Here's how the part is built. I have some questions about the finished solid (model axes, mm). A direction names the side the tool comes from. Give positions to 0.01 mm unless a question says otherwise; leave off trailing zeros.
from build123d import *

# Parameters (mm, degrees)
SKETCH1_R           = 2.5
BOSS_EXTRUDE1_DEPTH = 13.97
CUT_EXTRUDE1_REACH  = 108.146
SKETCH2_R           = 2.5
FILLET1_R           = 5
FILLET2_R           = 1


with BuildPart() as part:
    # Sketch1 → Boss-Extrude1 (new body)
    with BuildSketch(Plane(origin=(0, 0, 0), x_dir=(1, 0, 0), z_dir=(0, 1, 0))):
        Polygon((0, 7.071067812), (-7.071067812, 0), (62.778932188, -69.85), (81.2, -69.85), (81.2, -59.85), (66.921067812, -59.85), align=None)
        with Locations(Location((0, 0, 0), (0, 0, 270))):
            Circle(SKETCH1_R, mode=Mode.SUBTRACT)
    extrude(amount=BOSS_EXTRUDE1_DEPTH)

    # Sketch2 → Cut-Extrude1 (cut, up to next)
    with BuildSketch(Plane(origin=(0, 0, 59.85), x_dir=(-1, 0, 0), z_dir=(0, 0, -1)), mode=Mode.PRIVATE) as cut_extrude1_sk1:
        with Locations((-76.2, 7.62)):
            Circle(SKETCH2_R)
    cut_extrude1_tool1 = extrude(cut_extrude1_sk1.sketch, amount=-CUT_EXTRUDE1_REACH, mode=Mode.PRIVATE) & part.part
    add(cut_extrude1_tool1.solids().sort_by_distance((76.2, 7.62, 59.85))[0], mode=Mode.SUBTRACT)

    # Fillet1
    fillet1_edges = [part.edges().sort_by_distance(p)[0] for p in [
        (0, 6.985, -7.071067812),
        (-7.071067812, 6.985, 0),
        (81.2, 0, 64.85),
        (81.2, 13.97, 64.85),
        (62.778932188, 6.985, 69.85),
        (66.921067812, 6.985, 59.85),
    ]]
    fillet(fillet1_edges, radius=FILLET1_R - 0.0001)  # a hair under: the kernel refuses the full size

    # Fillet2
    fillet2_edges = [part.edges().sort_by_distance(p)[0] for p in [
        (70.525029289, 0, 69.85),
        (28.889445383, 0, 35.960513195),
        (34.496047101, 0, 27.424979289),
        (72.596097101, 0, 59.85),
        (62.936579685, 0, 69.469405275),
        (-5.000041421, 0, 0),
        (0, 0, -5.000041421),
        (34.496047101, 13.97, 27.424979289),
        (72.596097101, 13.97, 59.85),
        (28.889445383, 13.97, 35.960513195),
        (70.525029289, 13.97, 69.85),
        (62.936579685, 13.97, 69.469405275),
        (-5.000041421, 13.97, 0),
        (0, 13.97, -5.000041421),
        (81.2, 6.985, 59.85),
        (81.2, 6.985, 69.85),
        (79.735563195, 12.505563195, 59.85),
        (79.735563195, 1.464436805, 59.85),
        (79.735563195, 12.505563195, 69.85),
        (79.735563195, 1.464436805, 69.85),
        (67.078715309, 0, 59.469405275),
        (67.078715309, 13.97, 59.469405275),
    ]]
    fillet(fillet2_edges, radius=FILLET2_R)


solid = part.part
Q1. For faces 1 (the face through (73, 7, 59.85)), 2 (the face through (78.184, 6.099, 64.78)), which set-ups out of +Z, -Z, +X, -X, +Y, -Y let a thin tool reach every point of the face, with its end or its side?
Filled sheet:
face 1: -Z, +X, +Y, -Y
face 2: +Z, -Z
Q2. I need wall thicknesses on L1, parallel to Y at x = 76.2, z = 63.75; L2, parallel to X at y = 8.5, z = 60; L3, parallel to Z at x = 73, y = 2. Which ranges of each line are inside material? Lowest first, please.
Filled sheet:
L1: y = 0 to 5.12, 10.12 to 13.97
L2: x = 52.93 to 73.86, 78.54 to 80.73
L3: z = 59.85 to 69.85
Q3. Thinking about a two-plate mould opening in Z: for faces 3 (the face through (-5, 7, 0)), 4 (the face through (-2.44, 6.89, -0.54)), 5 (the face through (81.2, 7, 65)), which applies, released by +Z, released by -Z, zero draft, split by the parting line, or undercut?
Filled sheet:
face 3: split by the parting line
face 4: undercut
face 5: zero draft
Q4. I'm going to push flat-ended pins straight in: P1, Ø4, axis at x = 56.5, y = 4, coming from the -Z side; P2, Ø10, axis at x = 62.5, z = 43, coming from the +Y side; P3, Ø8, axis at x = 65, y = 2, coming from the -Z side; P4, Ø8, axis at y = 2, z = 13.5, coming from the -X side. Where does each tip first touch, or does it pass through?
Filled sheet:
P1: stops at z = 47.43
P2: passes through
P3: stops at z = 53.93
P4: stops at x = 2.43
Q5. If we section it at A-A on y = 7.62: Give the number of separate pieces and of enclosed holes in the cut face, plus the area to 3 significant figures.
Filled sheet:
separate pieces: 2
enclosed holes: 1
area: 1,050 mm2
